Geometry: final body of the model. Coordinates: model frame, mm. Face numbers are marked on the shaded views. A direction names the side the tool comes from. Coordinates: 2 decimals unless noted, no trailing zeros. Write each loop counter-clockwise with the first axis right and the second up, starting at its lowest first coordinate (ties: lowest second). Pieces come first, ordered by that corner, then holes.
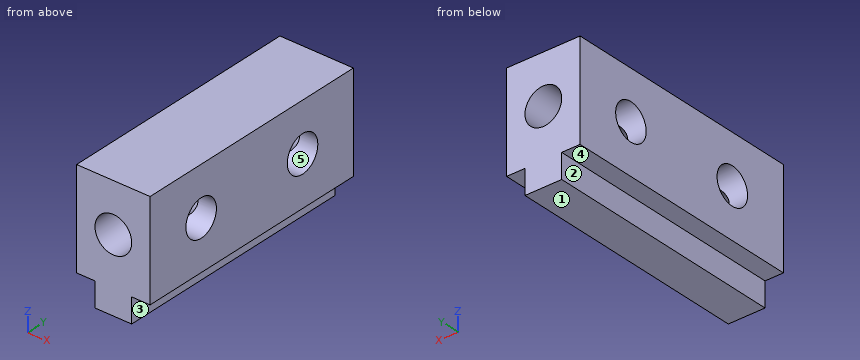
from build123d import *

# Parameters (mm, degrees)
F0_R     = 9.525
F1_DEPTH = 127
F2_R     = 9.525
F3_DEPTH = 129.794
F4_DEPTH = 104.14


with BuildPart() as f1:
    # F0 (on Front) → F1 (new body)
    with BuildSketch(Plane.XZ):
        Polygon((-14.114713, 40.939018), (-52.214713, 40.939018), (-52.214713, 15.539018), (-52.214713, -9.860982), (-42.689713, -9.860982), (-42.689713, -22.560982), (-23.639713, -22.560982), (-23.639713, -9.860982), (-14.114713, -9.860982), align=None)
        with Locations((-33.164713, 15.539018)):
            Circle(F0_R, mode=Mode.SUBTRACT)
    extrude(amount=F1_DEPTH)

    # F2 (on Right) → F3 (cut)
    with BuildSketch(Plane.YZ):
        with Locations((-95.083439, 15.739672)):
            Circle(F2_R)
    extrude(amount=-F3_DEPTH, mode=Mode.SUBTRACT)

    # F2 (on Right) → F4 (cut)
    with BuildSketch(Plane.YZ):
        with Locations((-31.75, 15.739672)):
            Circle(F2_R)
    extrude(amount=-F4_DEPTH, mode=Mode.SUBTRACT)


solid = f1.part
Item 1: Set-up query: the marked faces 1 and 2. Return all of +Z, -Z, +X, -X, +Y, -Y with unobstructed straight access to the full face (end or side cutting, diameter ignored); none if empty.
Derived:
face 1: -Z, +X, -X, +Y, -Y
face 2: -Z, -X, +Y, -Y
Item 2: Pull-direction query (Z, two-part tool) for the marked faces 3, 4 and 5; classes: released by +Z, released by -Z, zero draft, split by the parting line, or undercut.
Derived:
face 3: zero draft
face 4: released by -Z
face 5: undercut
Item 3: Pin query (flat end, axial travel): pin 1 (5 mm diameter, centred on x = -19, y = -57.5, fed in from -Z); pin 2 (6.5 mm diameter, centred on y = -62, z = -18, fed in from +X); pin 3 (10 mm diameter, centred on x = -26, z = 17.5, fed in from -Y). Return the tip coordinate at first contact, or that it passes through.
Derived:
pin 1: stops at z = -9.86
pin 2: stops at x = -23.64
pin 3: stops at y = -127
Item 4: Section D-D, the plane y = -15.5. Output: boundary loops of the cut face in (x, z) (3 decimals), plus the area to 3 significant figures.
Derived:
outline: (-52.215, -9.861) - (-42.69, -9.861) - (-42.69, -22.561) - (-23.64, -22.561) - (-23.64, -9.861) - (-14.115, -9.861) - (-14.115, 40.939) - (-52.215, 40.939) - close; hole circle Ø19.05 at (-33.165, 15.539)
area: 1,890 mm2
Item 5: Material intervals for probe 1 along Y at (x, z) = (-21.5, 24); probe 2 along Y at (x, z) = (-51, 14); probe 3 along X at (y, z) = (-61.5, -10.5), sorted ascending.
Derived:
probe 1: y = -127 to -99.83, -90.34 to -36.49, -27.01 to 0
probe 2: y = -127 to -104.45, -85.72 to -41.11, -22.39 to 0
probe 3: x = -42.69 to -23.64
Item 6: Section C-C, the plane x = -25. Output: boundary loops of the cut face in (y, z) (3 decimals).
Derived:
outline: (-127, -22.561) - (0, -22.561) - (0, 10.634) - (-23.709, 10.634) arc R9.525 cw to (-39.791, 10.634) - (-87.043, 10.634) arc R9.525 cw to (-103.124, 10.634) - (-127, 10.634) - close; (-127, 20.444) - (-103.365, 20.444) arc R9.525 cw to (-86.801, 20.444) - (-40.032, 20.444) arc R9.525 cw to (-23.468, 20.444) - (0, 20.444) - (0, 40.939) - (-127, 40.939) - close
Item 7: Section A-A, the plane z = 11. Output: boundary loops of the cut face in (x, y), plus the area to 3 significant figures.
Derived:
outline: (-52.21, -127) - (-41.54, -127) - (-41.54, -103.35) - (-52.21, -103.35) - close; (-52.21, -86.82) - (-41.54, -86.82) - (-41.54, -40.01) - (-52.21, -40.01) - close; (-52.21, -23.49) - (-41.54, -23.49) - (-41.54, 0) - (-52.21, 0) - close; (-24.79, -127) - (-14.11, -127) - (-14.11, -103.35) - (-24.79, -103.35) - close; (-24.79, -86.82) - (-14.11, -86.82) - (-14.11, -40.01) - (-24.79, -40.01) - close; (-24.79, -23.49) - (-14.11, -23.49) - (-14.11, 0) - (-24.79, 0) - close
area: 2,010 mm2
